```python
from build123d import *

# Parameters (mm, degrees)
SKETCH1_W           = 0.4
SKETCH1_H           = 4
SKETCH1_W_2         = 4
SKETCH1_H_2         = 3
BOSS_EXTRUDE1_DEPTH = 0.2
BOSS_EXTRUDE3_START = -0.2
BOSS_EXTRUDE3_DEPTH = 0.200006


with BuildPart() as part:
    # Sketch1 → Boss-Extrude1 (new body)
    with BuildSketch(Plane(origin=(0, 0, 0), x_dir=(1, 0, 0), z_dir=(0, 1, 0))):
        with Locations((3.376311417, -1.321333446)):
            Rectangle(SKETCH1_W, SKETCH1_H)
        with Locations((3.379701823, 2.178666554)):
            Rectangle(SKETCH1_W_2, SKETCH1_H_2)
    extrude(amount=BOSS_EXTRUDE1_DEPTH)

    # Sketch5 → Boss-Extrude3 (add)
    with BuildSketch(Plane(origin=(0, 0.2, 0), x_dir=(1, 0, 0), z_dir=(0, 1, 0)).offset(BOSS_EXTRUDE3_START)):
        Polygon((3.176311417, -3.321333446), (3.576311417, -3.321333446), (3.376311417, -4.295422221), align=None)
    extrude(amount=BOSS_EXTRUDE3_DEPTH)


solid = part.part
```
Geometry check sheet. Reference: the model listing, model coordinates, mm. Coordinates: 2 decimals unless noted, no trailing zeros. Write each loop counter-clockwise with the first axis right and the second up, starting at its lowest first coordinate (ties: lowest second). Pieces come first, ordered by that corner, then holes. Notation, with made-up numbers: M -21.5,50 L 19.5,50 A29 cw 19.5,75 Z; hole C -37,-5 d9. An arc over 180 degrees is marked long. One line per item, written item: value. Start each with the question number.
(1) Sectioned sample at A-A, the plane y = 0.15. Enter the section's corners in (x, z).
(2) Scan lines: line 1 along Z through (x, y) = (4.85, 0.1); line 2 along X through (y, z) = (0.15, 1); line 3 along X through (y, z) = (0.1, 3.5). Record each from-to range of solid material in increasing order. Write a range as [from, to].
(3) Sectioned sample at C-C, the plane x = 4.7. Enter the section's corners in (y, z), and give its area (3 significant figures).
(4) Depth check by flat-ended pin: pin 1 (1.5 mm diameter, centred on x = 3.5, z = -2.5, fed in from -Y). Enter the tip coordinate at first touch or a pass-through.
(5) Sectioned sample at B-B, the plane z = 0.75. Enter the section's corners in (x, y), and give its area (3 significant figures).
Filled sheet:
1. outline: M 1.38,-3.68 L 5.38,-3.68 L 5.38,-0.68 L 3.58,-0.68 L 3.58,3.32 L 3.38,4.3 L 3.18,3.32 L 3.18,-0.68 L 1.38,-0.68 Z
2. line 1: [-3.68, -0.68]
2. line 2: [3.18, 3.58]
2. line 3: [3.21, 3.54]
3. outline: M 0,-3.68 L 0.2,-3.68 L 0.2,-0.68 L 0,-0.68 Z
3. area: 0.600 mm²
4. pin 1: y = 0
5. outline: M 3.18,0 L 3.58,0 L 3.58,0.2 L 3.18,0.2 Z
5. area: 0.0800 mm²
